Drawing for the job (mm, zero at the part's lowest x, y, z). Coordinates: 2 decimals unless noted, no trailing zeros. Order: outer loops, then holes, each group sorted by start corner. A loop starts at its lowest first (then second) coordinate and runs counter-clockwise, first axis right, second up.
1) Cut at A-A (z = 12.5). List the corners of the cut face in (x, y), and give its area (3 significant figures).
2) Mould opens along Z. For the marked faces 1, 2, 3 and 4 say: +Z half, -Z half, draft (parallel to the pull), parting line (faces both ways), or undercut.
3) Wall check: L1, parallel to Y at x = 1.8, z = 15.5; L2, parallel to Y at x = 1.95, z = 10; L3, parallel to Y at x = 1.1, z = 3. Give the ranges that are in metal, low to high.
4) Cut at D-D (y = 20.25). List the corners of the cut face in (x, z), and give its area (3 significant figures).
5) Cut at B-B (x = 1.35). List the corners of the cut face in (y, z), and give its area (3 significant figures).
6) Cut at C-C (z = 20.25). List the corners of the cut face in (x, y).
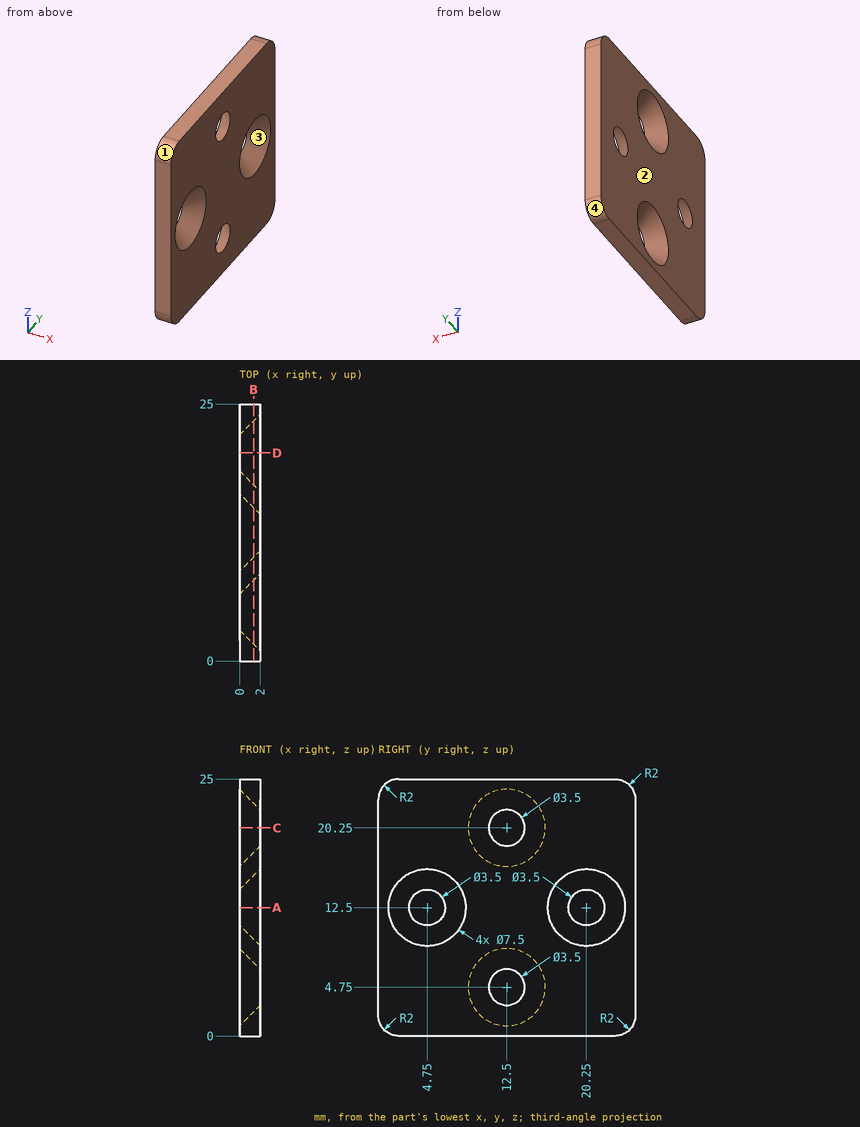
Geometry check:
1. outline: (0, 0) - (2, 0) - (2, 1) - (0, 3) - close; (0, 6.5) - (2, 8.5) - (2, 16.5) - (0, 18.5) - close; (0, 22) - (2, 24) - (2, 25) - (0, 25) - close
1. area: 28.0 mm2
2. face 1: +Z half
2. face 2: draft
2. face 3: undercut
2. face 4: -Z half
3. L1: y = 0 to 2.85, 6.65 to 18.35, 22.15 to 25
3. L2: y = 0 to 2.02, 7.48 to 17.52, 22.98 to 25
3. L3: y = 0 to 10.51, 14.49 to 25
4. outline: (0, 0) - (2, 0) - (2, 8.75) - (0, 10.75) - close; (0, 14.25) - (2, 16.25) - (2, 25) - (0, 25) - close
4. area: 39.0 mm2
5. outline: (0, 2) arc R2 ccw to (2, 0) - (23, 0) arc R2 ccw to (25, 2) - (25, 23) arc R2 ccw to (23, 25) - (2, 25) arc R2 ccw to (0, 23) - close; hole circle Ø6.2 at (4.75, 12.5); hole circle Ø4.8 at (12.5, 4.75); hole circle Ø4.8 at (12.5, 20.25); hole circle Ø6.2 at (20.25, 12.5)
5. area: 525 mm2
6. outline: (0, 0) - (2, 0) - (2, 10.75) - (0, 8.75) - close; (0, 16.25) - (2, 14.25) - (2, 25) - (0, 25) - close
